Can you work these out from the drawing? Everything is in mm from the part's minimum corner. A direction names the side the tool comes from. Coordinates: 2 decimals unless noted, no trailing zeros. Loops run counter-clockwise (first coordinate to the right, second up) from the corner with the lowest first, then second, coordinate; pieces in that order, holes last.
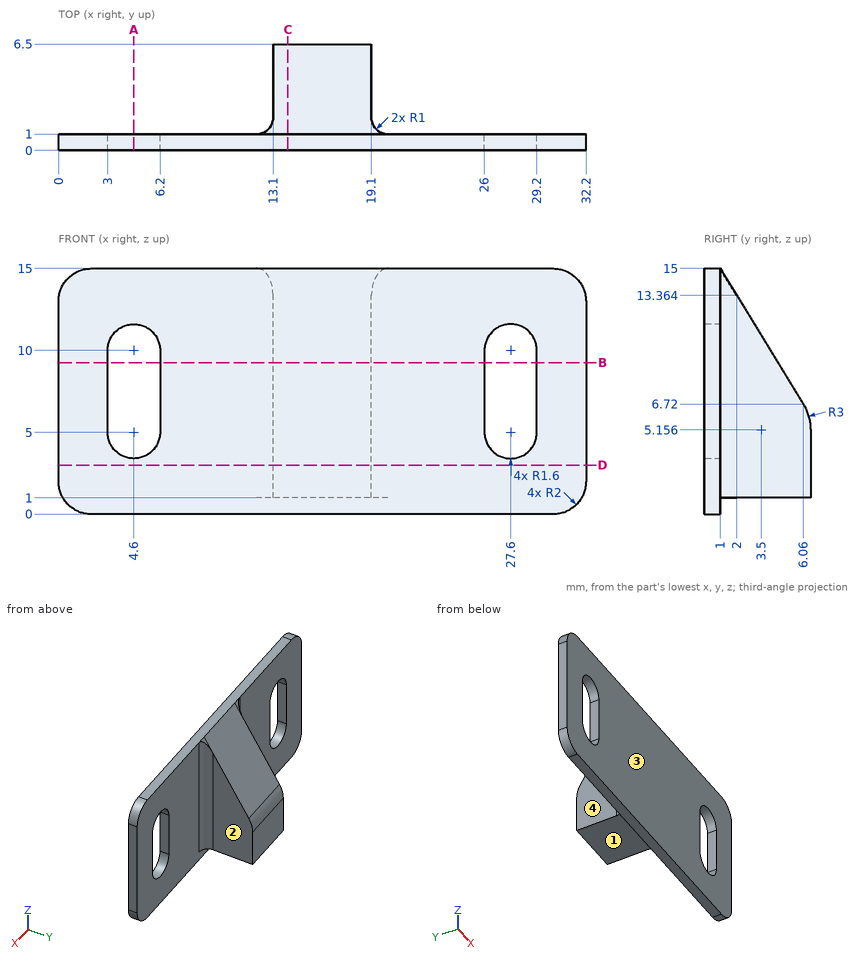
1. I want a section at A-A (x = 4.6). Please give me the cut outline in (y, z).
2. For pin 1 (2 mm diameter, centred on y = 4, z = 9, fed in from +X); pin 2 (1.6 mm diameter, centred on x = 14.5, y = 2.5, fed in from -Z); pin 3 (3.5 mm diameter, centred on y = 5, z = 8, fed in from -X), each with a flat end and sliding along its axis, tell me the tip position at first contact or that it passes through.
3. I want a section at B-B (z = 9.25). Please give me the cut outline in (x, y).
4. I need wall thicknesses on line 1 along X through (y, z) = (0.5, 11); line 2 along X through (y, z) = (5.75, 3); line 3 along Y through (x, z) = (12, 3). Which ranges of each line are inside material? Lowest first, please.
5. I want a section at D-D (z = 3). Please give me the cut outline in (x, y).
6. I want a section at C-C (x = 14). Please give me the cut outline in (y, z), then the cut area to 3 significant figures.
7. On a 3-axis mill with a long thin cutter (end or side, diameter ignored), from which of +Z, -Z, +X, -X, +Y, -Y can I reach the whole of each face in a straight line? I mean the marked faces 1, 2, 3 and 4. Say none if no direction works.
Response values:
1. outline: (0, 0) - (1, 0) - (1, 3.4) - (0, 3.4) - close; (0, 11.6) - (1, 11.6) - (1, 15) - (0, 15) - close
2. pin 1: stops at x = 19.1
2. pin 2: stops at z = 1
2. pin 3: stops at x = 13.1
3. outline: (0, 0) - (3, 0) - (3, 1) - (0, 1) - close; (6.2, 0) - (26, 0) - (26, 1) - (20.1, 1) arc R1 cw to (19.1, 2) - (19.1, 4.51) - (13.1, 4.51) - (13.1, 2) arc R1 cw to (12.1, 1) - (6.2, 1) - close; (29.2, 0) - (32.2, 0) - (32.2, 1) - (29.2, 1) - close
4. line 1: x = 0 to 3.35, 5.85 to 26.35, 28.85 to 32.2
4. line 2: x = 13.1 to 19.1
4. line 3: y = 0 to 1
5. outline: (0, 0) - (32.2, 0) - (32.2, 1) - (20.1, 1) arc R1 cw to (19.1, 2) - (19.1, 6.5) - (13.1, 6.5) - (13.1, 2) arc R1 cw to (12.1, 1) - (0, 1) - close
6. outline: (0, 0) - (1, 0) - (1, 1) - (6.5, 1) - (6.5, 5.16) arc R3 ccw to (6.06, 6.72) - (1, 15) - (0, 15) - close
6. area: 67.2 mm2
7. face 1: -Z, +X, -X, +Y
7. face 2: +Z, -Z, +X, +Y
7. face 3: +Z, -Z, +X, -X, -Y
7. face 4: +Z, -Z, -X, +Y
